Read the model definition and answer for the solid it produces. Units are mm, in the model's axes. A direction names the side the tool comes from. Give positions to 0.01 mm unless a question says otherwise; leave off trailing zeros. Loops run counter-clockwise (first coordinate to the right, second up) from the corner with the lowest first, then second, coordinate; pieces in that order, holes last. Notation, with made-up numbers: (-38, 82) - (12, 82) arc R29 ccw to (12, 112) - close; hole circle Ø9 at (21, -7). An arc over 180 degrees is marked (long way). Put each result on its own line as item: value. Start each with the question number.
1. A cutting plane is placed at C-C, the plane y = 7.25. Determine the outline of the cut face in (x, z), plus the area to 3 significant figures.
2. For faces 1 (the flat face through (0, 16, 0)), 2 (the cylindrical face through (1.437, 7.642, -1.318)), 3 (the cylindrical face through (1.437, -4.219, 1.318)), determine the directions among +Z, -Z, +X, -X, +Y, -Y from which every point of the face is accessible in a straight line to the end or side of a thin tool.
3. Given pin 1 Ø2 at (x, y) = (-2, -0.5) entering from +Z; pin 2 Ø1.5 at (y, z) = (-3, -1) entering from +X; pin 3 Ø1.5 at (y, z) = (12.5, 0.5) entering from -X, each flat-ended and moving along its own axis, determine where each tip first touches the part or whether it passes through.
4. A cutting plane is placed at B-B, the plane x = 0. Determine the outline of the cut face in (y, z).
5. A cutting plane is placed at A-A, the plane z = 0. Determine the outline of the cut face in (x, y).
6. Consider L1, parallel to Y at x = -2.5, z = 0; L2, parallel to Z at x = 1, y = 7.5; L3, parallel to X at y = 6, z = 1.25. Determine where each line is inside the solid, lowest interval first. Write a range as from..to.
Autodesk Inventor part; units mm, degrees
ref_plane "YZ Plane" through (0, 0, 0) normal (1, 0, 0) x (0, 1, 0)
ref_plane "XZ Plane" through (0, 0, 0) normal (0, 1, 0) x (-1, 0, 0)
ref_plane "XY Plane" through (0, 0, 0) normal (0, 0, 1) x (1, 0, 0)
sketch "Sketch1" plane through (0, 0, 0) normal (0, 1, 0) x (-1, 0, 0)
  circle A0 centre (0, 0) radius 1.95
  dimension "d0" = 3.9
extrude "Extrusion1" add sketch "Sketch1" along normal blind 16 and the other way blind 7
sketch "Sketch2" plane through (0, 0, 0) normal (0, 1, 0) x (-1, 0, 0)
  circle A0 centre (0, 0) radius 1.95
  circle A1 centre (0, 0) radius 3.45
  dimension "d5" = 1.5
extrude "Extrusion2" add sketch "Sketch2" against normal blind 2
chamfer "Chamfer1" distance 0.5 angle 45 3 edges at (1.95, 16, 0) (1.95, -7, 0) (3.45, -2, 0)
properties part number "button"
Return value:
1. outline: circle Ø3.9 at (0, 0)
1. area: 11.9 mm2
2. face 1: +Z, -Z, +X, -X, +Y
2. face 2: +Y
2. face 3: -Y
3. pin 1: stops at z = 3.3
3. pin 2: stops at x = 1.93
3. pin 3: stops at x = -1.95
4. outline: (-7, -1.45) - (-6.5, -1.95) - (-2, -1.95) - (-2, -2.95) - (-1.5, -3.45) - (0, -3.45) - (0, -1.95) - (15.5, -1.95) - (16, -1.45) - (16, 1.45) - (15.5, 1.95) - (0, 1.95) - (0, 3.45) - (-1.5, 3.45) - (-2, 2.95) - (-2, 1.95) - (-6.5, 1.95) - (-7, 1.45) - close
5. outline: (-3.45, -1.5) - (-2.95, -2) - (-1.95, -2) - (-1.95, -6.5) - (-1.45, -7) - (1.45, -7) - (1.95, -6.5) - (1.95, -2) - (2.95, -2) - (3.45, -1.5) - (3.45, 0) - (1.95, 0) - (1.95, 15.5) - (1.45, 16) - (-1.45, 16) - (-1.95, 15.5) - (-1.95, 0) - (-3.45, 0) - close
6. L1: y = -2..0
6. L2: z = -1.67..1.67
6. L3: x = -1.5..1.5
